Read the model definition and answer for the solid it produces. Units are mm, in the model's axes. A direction names the side the tool comes from. Coordinates: 2 decimals unless noted, no trailing zeros. Loops run counter-clockwise (first coordinate to the right, second up) from the corner with the lowest first, then second, coordinate; pieces in that order, holes last. Notation, with made-up numbers: (35, 21.5) - (88, 21.5) arc R10 ccw to (88, 37.5) - close; hole circle Ø10 at (61, 80). An arc over 180 degrees is marked (long way). Use CSV: the item, a comma, the result in double quotes.
```python
from build123d import *

# Parameters (mm, degrees)
BASE_FLANGE1_DEPTH = 100
SKETCH6_R          = 4
CUT_EXTRUDE1_DEPTH = 10


# Sheet-metal steps are written as plain solids
with BuildPart() as part:
    # Sketch1 → Base-Flange1 (new body)
    with BuildSketch(Plane.XY):
        with BuildLine():
            Line((0, 300), (0, 0.7366))
            ThreePointArc((0, 0.7366), (0.215745145, 0.215745145), (0.7366, 0))
            Line((0.7366, 0), (200, 0))
            Line((200, 0), (200, -0.7366))
            Line((200, -0.7366), (0.7366, -0.7366))
            ThreePointArc((0.7366, -0.7366), (-0.30510971, -0.30510971), (-0.7366, 0.7366))
            Line((-0.7366, 0.7366), (-0.7366, 300))
            Line((-0.7366, 300), (0, 300))
        make_face()
    extrude(amount=BASE_FLANGE1_DEPTH)

    # Sketch6 → Cut-Extrude1 (cut)
    with BuildSketch(Plane(origin=(0, 0, 0), x_dir=(1, 0, 0), z_dir=(0, 1, 0))):
        with Locations(Location((170, -15, 0), (0, 0, 270))):
            Circle(SKETCH6_R)
        with Locations(Location((170, -85, 0), (0, 0, 270))):
            Circle(SKETCH6_R)
    extrude(amount=-CUT_EXTRUDE1_DEPTH, mode=Mode.SUBTRACT)


solid = part.part
```
Q1. The part is cut by section D-D on x = 12. Determine the outline of the cut face in (y, z), and give its area (3 significant figures).
Reported:
outline,"(-0.74, 0) - (0, 0) - (0, 100) - (-0.74, 100) - close"
area,"73.7 mm²"
Q2. The part is cut by section C-C on z = 37. Determine the outline of the cut face in (x, y), and give its area (3 significant figures).
Reported:
outline,"(-0.74, 0.74) arc R1.47 ccw to (0.74, -0.74) - (200, -0.74) - (200, 0) - (0.74, 0) arc R0.74 cw to (0, 0.74) - (0, 300) - (-0.74, 300) - close"
area,"368 mm²"
Q3. The part is cut by section A-A on x = 170. Determine the outline of the cut face in (y, z), and give its area (3 significant figures).
Reported:
outline,"(-0.74, 0) - (0, 0) - (0, 11) - (-0.74, 11) - close; (-0.74, 19) - (0, 19) - (0, 81) - (-0.74, 81) - close; (-0.74, 89) - (0, 89) - (0, 100) - (-0.74, 100) - close"
area,"61.9 mm²"
Q4. Find the intervals of material crossed by probe 1 along X at (y, z) = (-0.5, 85); probe 2 along Y at (x, z) = (94, 87.5), in increasing order. Write a range as [from, to].
Reported:
probe 1,"x = [-0.06, 166], [174, 200]"
probe 2,"y = [-0.74, 0]"
Q5. Given P1, Ø3, axis at y = 76, z = 54, coming from the +X side, flat-ended and moving along its own axis, determine where the tip first touches the part or whether it passes through.
Reported:
P1,"stops at x = 0"
Q6. For a pull along X with two mould halves and no side action, classify faces 3 (the face through (99, 0, 49)), 4 (the face through (-0.737, 148, 49)), 5 (the face through (173.966, -0.363, 14.479)) as +X half, -X half, draft (parallel to the pull), parting line (faces both ways), or undercut.
Reported:
face 3,"draft"
face 4,"-X half"
face 5,"undercut"
Q7. The part is cut by section B-B on z = 85. Determine the outline of the cut face in (x, y), and give its area (3 significant figures).
Reported:
outline,"(-0.74, 0.74) arc R1.47 ccw to (0.74, -0.74) - (166, -0.74) - (166, 0) - (0.74, 0) arc R0.74 cw to (0, 0.74) - (0, 300) - (-0.74, 300) - close; (174, -0.74) - (200, -0.74) - (200, 0) - (174, 0) - close"
area,"363 mm²"
Q8. A tool of negligible diameter and unlimited length cuts with its end or side. For faces 1 (the face through (173.966, -0.363, 84.479)), 2 (the face through (0, 152, 49)), from which of +Z, -Z, +X, -X, +Y, -Y can it reach the whole face along a straight path? Write none if from no direction.
Reported:
face 1,"+Y, -Y"
face 2,"+Z, -Z, +X, +Y"
